Could you check a few things on this drawing? It's one solid part, dimensions in mm from its lowest x, y, z. Give positions to 0.01 mm unless a question says otherwise; leave off trailing zeros. Order: outer loops, then holes, each group sorted by start corner. A loop starts at its lowest first (then second) coordinate and runs counter-clockwise, first axis right, second up.
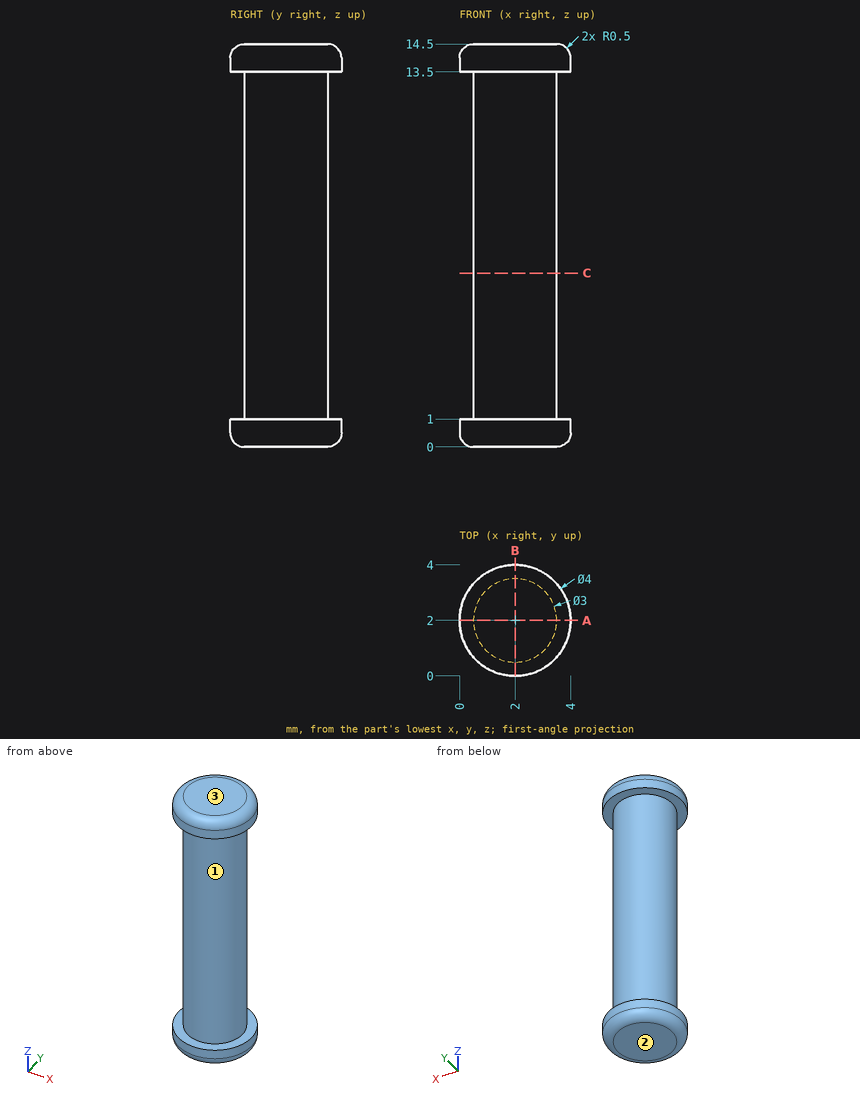
Item 1: Imagine slicing it at A-A on y = 2. List the corners of the cut face in (x, z) for me.
Findings:
outline: (0, 0.5) arc R0.5 ccw to (0.5, 0) - (3.5, 0) arc R0.5 ccw to (4, 0.5) - (4, 1) - (3.5, 1) - (3.5, 13.5) - (4, 13.5) - (4, 14) arc R0.5 ccw to (3.5, 14.5) - (0.5, 14.5) arc R0.5 ccw to (0, 14) - (0, 13.5) - (0.5, 13.5) - (0.5, 1) - (0, 1) - close
Item 2: We'd pull the mould along Z, two halves only. Please class the marked faces 1, 2 and 3: +Z half, -Z half, draft (parallel to the pull), parting line (faces both ways), or undercut.
Findings:
face 1: undercut
face 2: -Z half
face 3: +Z half
Item 3: For pin 1 (1.2 mm diameter, centred on x = 2, y = 2, fed in from -Z); pin 2 (1 mm diameter, centred on x = 2.5, z = 12.5, fed in from +Y), each with a flat end and sliding along its axis, tell me the tip position at first contact or that it passes through.
Findings:
pin 1: stops at z = 0
pin 2: stops at y = 3.5
Item 4: Please list where these lines run through material, in increasing order: line 1 along X through (y, z) = (1.9, 5.25); line 2 along Z through (x, y) = (3.6, 3).
Findings:
line 1: x = 0.5 to 3.5
line 2: z = 0.18 to 1, 13.5 to 14.32
Item 5: Imagine slicing it at C-C on z = 6.25. List the corners of the cut face in (x, y) for me, then the cut area to 3 significant figures.
Findings:
outline: circle Ø3 at (2, 2)
area: 7.07 mm2
